Geometry: final body of the model. Coordinates: model frame, mm. Give positions to 0.01 mm unless a question says otherwise; leave off trailing zeros. Write each loop counter-clockwise with the first axis right and the second up, starting at its lowest first coordinate (ties: lowest second). Pieces come first, ordered by that corner, then holes.
Q1. Line query: L1, parallel to X at y = 29, z = 11; L2, parallel to X at y = 31, z = 6; L3, parallel to Y at x = 1, z = 29.5. Output: solid intervals per line, ascending.
Q2. Cut plane D-D on z = 18. Return the cut outline in (x, y), plus the area to 3 significant figures.
Q3. Cut plane B-B on y = 25.5. Return the cut outline in (x, z).
Q4. Cut plane A-A on y = 55. Return the cut outline in (x, z), plus the area to 3 significant figures.
Q5. Cut plane C-C on x = 62. Return the cut outline in (y, z), plus the area to 3 significant figures.
Q6. Pin query (flat end, axial travel): pin 1 (5 mm diameter, centred on x = -45, y = 55.5, fed in from -Z); pin 2 (5 mm diameter, centred on y = 19.5, z = 10, fed in from -X); pin 3 (1.5 mm diameter, centred on x = -7, z = 31.5, fed in from -Y); pin 4 (5 mm diameter, centred on y = 56, z = 9, fed in from -X). Return the tip coordinate at first contact, or that it passes through.
Q7. Draft query along Z for faces 1 (the face through (0, 84, 0)), 2 (the face through (0, 91, 2.54)). Return one class per face: pulls with the +Z half, pulls with the -Z half, needs draft (parallel to the pull), parting line crosses it, or undercut.
```python
from build123d import *

# Parameters (mm, degrees)
F1_ANGLE      = 30
F2_R          = 3.81
F3_DEPTH      = 87.631
F3_DEPTH_BACK = 87.631
F4_W          = 5.08
F4_H          = 7.62
F5_DEPTH      = 2.54


with BuildPart() as f1:
    # F0 (on Top) → F1 (revolve)
    with BuildSketch(Plane.XY):
        with BuildLine():
            Line((-87.63, 0), (-82.55, 0))
            ThreePointArc((-82.55, 0), (0, 82.55), (82.55, 0))
            Line((82.55, 0), (87.63, 0))
            ThreePointArc((87.63, 0), (0, 87.63), (-87.63, 0))
        make_face()
    revolve(axis=Axis((-41.275, 0, 0), (1, 0, 0)), revolution_arc=F1_ANGLE)

    # F2 (on Right) → F3 (cut, two sides)
    with BuildSketch(Plane.YZ) as f3_sk:
        Circle(F2_R)
    extrude(amount=-F3_DEPTH, mode=Mode.SUBTRACT)
    extrude(f3_sk.sketch, amount=F3_DEPTH_BACK, mode=Mode.SUBTRACT)

    # F4 (on Top) → F5 (join)
    with BuildSketch(Plane.XY):
        with Locations((0, 91.4031806706)):
            Rectangle(F4_W, F4_H)
    extrude(amount=F5_DEPTH)


solid = f1.part
```
Data:
1. L1: x = -81.96 to -76.5, 76.5 to 81.96
1. L2: x = -81.74 to -76.27, 76.27 to 81.74
1. L3: y = 77.09 to 82.51
2. outline: (-79.89, 31.18) - (-74.29, 31.18) arc R80.56 cw to (74.29, 31.18) - (79.89, 31.18) arc R85.76 ccw to start
2. area: 1,030 mm2
3. outline: (-83.84, 0) - (-78.51, 0) arc R78.51 cw to (-77.12, 14.72) - (-82.53, 14.72) arc R83.84 ccw to start; (77.12, 14.72) arc R78.51 cw to (78.51, 0) - (83.84, 0) arc R83.84 ccw to (82.53, 14.72) - close
4. outline: (-68.22, 0) - (-61.56, 0) arc R61.56 cw to (-52.74, 31.75) - (-60.38, 31.75) arc R68.22 ccw to start; (52.74, 31.75) arc R61.56 cw to (61.56, 0) - (68.22, 0) arc R68.22 ccw to (60.38, 31.75) - close
4. area: 442 mm2
5. outline: (47.2, 27.25) arc R54.5 cw to (54.5, 0) - (61.93, 0) arc R61.93 ccw to (53.63, 30.96) - close
5. area: 226 mm2
6. pin 1: passes through
6. pin 2: stops at x = -85.45
6. pin 3: stops at y = 75.66
6. pin 4: stops at x = -68.84
7. face 1: pulls with the -Z half
7. face 2: pulls with the +Z half
